Answer from the drawing. Dimensions are ordinates in mm from the lowest x, y and z of the part. A direction names the side the tool comes from. Give positions to 0.01 mm unless a question says otherwise; leave off trailing zeros. Write each loop counter-clockwise with the first axis right and the second up, starting at its lowest first coordinate (ties: lowest second). Pieces come first, ordered by that corner, then holes. Notation, with made-up numbers: (-14, 83) -> (13, 83) arc R4 cw to (13, 88) -> close; hole circle Ø11 at (-17, -25). An arc over 180 degrees is marked (long way). Use a Markdown table: item, result. Add a question column.
Q1. For the marked faces 1 and 2, determine the directions among +Z, -Z, +X, -X, +Y, -Y from which every point of the face is accessible in a straight line to the end or side of a thin tool.
Q2. Consider line 1 (Y direction, x = 0.75, z = 9.5); line 2 (X direction, y = 1, z = 7); line 3 (Z direction, x = 15.25, y = 11). Determine where each line is inside the solid, lowest interval first.
Q3. Section D-D, the plane y = 15.25 is taken. Give the vertices of the cut face in (x, z).
Q4. Section A-A, the plane y = 9.5 is taken. Give the vertices of the cut face in (x, z).
Q5. Each of these flat-tipped pins is pushed along its axis until it touches: pin 1 Ø3.5 at (x, y) = (9, 9.5) entering from -Z; pin 2 Ø4 at (x, y) = (4.5, 9.5) entering from -Z. Where does it stop, or does it pass through?
Q6. Section B-B, the plane x = 9 is taken. Give the vertices of the cut face in (y, z).
Q7. Section C-C, the plane z = 9.5 is taken. Give the vertices of the cut face in (x, y), plus the area to 3 significant figures.
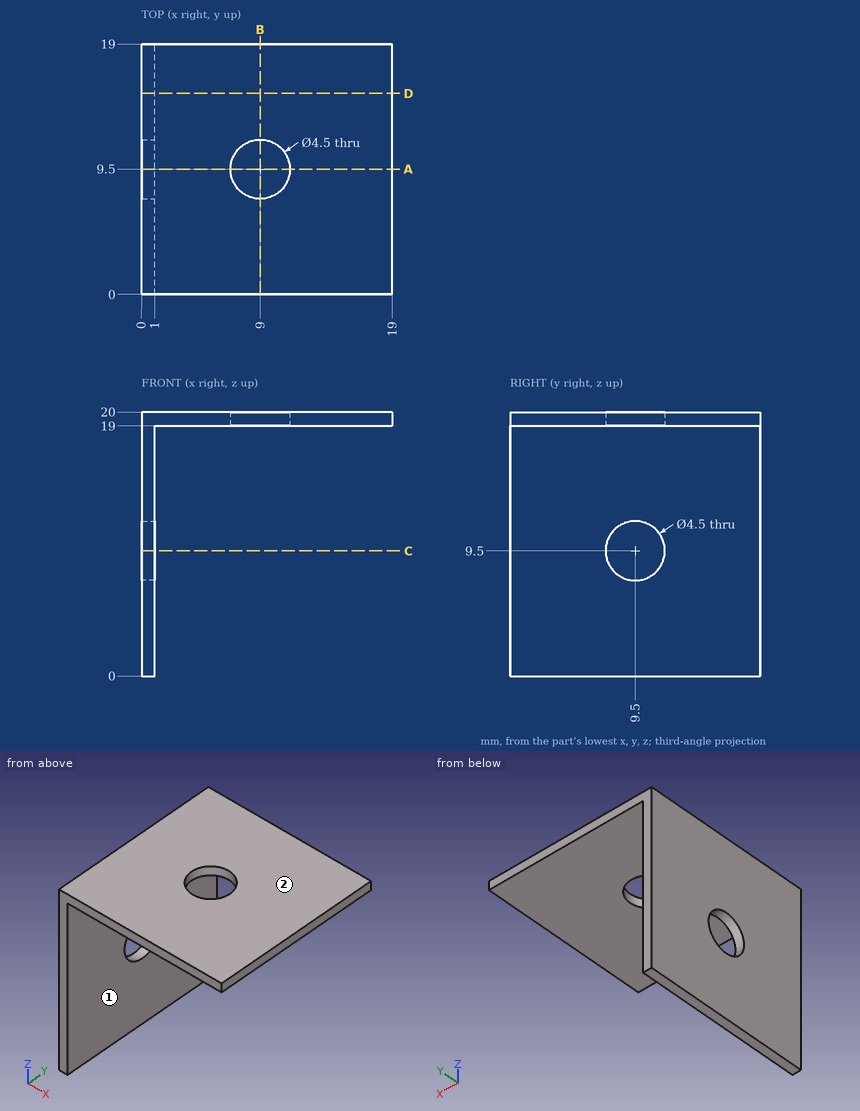
Result set:
| question | item | result |
|---|---|---|
| 1 | face 1 | -Z, +X, +Y, -Y |
| 1 | face 2 | +Z, +X, -X, +Y, -Y |
| 2 | line 1 | y = 0 to 7.25, 11.75 to 19 |
| 2 | line 2 | x = 0 to 1 |
| 2 | line 3 | z = 19 to 20 |
| 3 | outline | (0, 0) -> (1, 0) -> (1, 19) -> (19, 19) -> (19, 20) -> (0, 20) -> close |
| 4 | outline | (0, 0) -> (1, 0) -> (1, 7.25) -> (0, 7.25) -> close; (0, 11.75) -> (1, 11.75) -> (1, 19) -> (6.75, 19) -> (6.75, 20) -> (0, 20) -> close; (11.25, 19) -> (19, 19) -> (19, 20) -> (11.25, 20) -> close |
| 5 | pin 1 | passes through |
| 5 | pin 2 | stops at z = 19 |
| 6 | outline | (0, 19) -> (7.25, 19) -> (7.25, 20) -> (0, 20) -> close; (11.75, 19) -> (19, 19) -> (19, 20) -> (11.75, 20) -> close |
| 7 | outline | (0, 0) -> (1, 0) -> (1, 7.25) -> (0, 7.25) -> close; (0, 11.75) -> (1, 11.75) -> (1, 19) -> (0, 19) -> close |
| 7 | area | 14.5 mm2 |
